Can you work these out from the drawing? Everything is in mm from the part's minimum corner. A direction names the side the tool comes from. Give positions to 0.01 mm unless a question says otherwise; leave off trailing zeros. Order: outer loops, then holes, each group sorted by start corner. A loop starts at its lowest first (then second) coordinate and runs counter-clockwise, first axis right, second up. Notation, with made-up numbers: (9.25, 25.25) - (22.25, 25.25) arc R21 ccw to (22.25, 32.25) - close; hole circle Ø6 at (21.5, 23). An arc over 180 degrees is marked (long way). Answer as a JSON object with one key per item and string values.
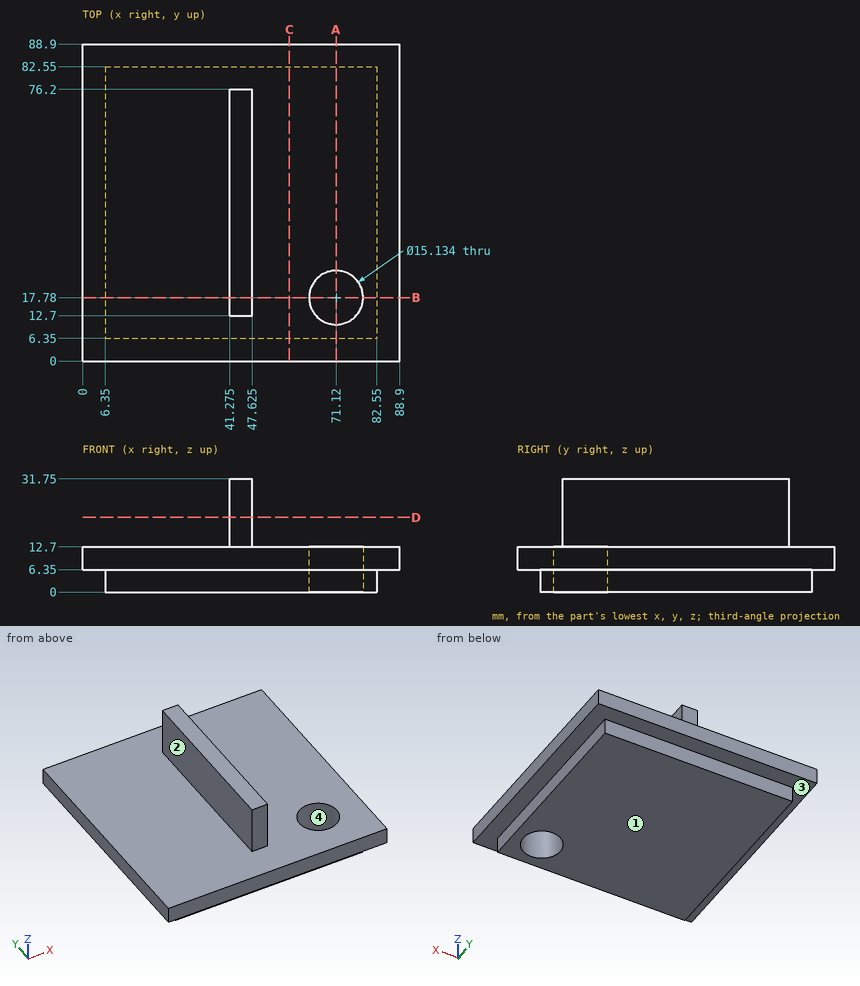
Q1. If we section it at B-B, the plane y = 17.78: Please give me the cut outline in (x, z) (3 decimals).
Recorded:
{"outline": "(0, 6.35) - (6.35, 6.35) - (6.35, 0) - (63.553, 0) - (63.553, 12.7) - (47.625, 12.7) - (47.625, 31.75) - (41.275, 31.75) - (41.275, 12.7) - (0, 12.7) - close; (78.687, 0) - (82.55, 0) - (82.55, 6.35) - (88.9, 6.35) - (88.9, 12.7) - (78.687, 12.7) - close"}
Q2. I'm going to push flat-ended pins straight in: pin 1 Ø1 at (y, z) = (14.5, 16.5) entering from -X (3 decimals); pin 2 Ø3 at (x, z) = (43, 17.5) entering from +Y; pin 3 Ø17.5 at (x, y) = (71.12, 17.78) entering from +Z. Where does each tip first touch, or does it pass through?
Recorded:
{"pin 1": "stops at x = 41.275", "pin 2": "stops at y = 76.2", "pin 3": "stops at z = 12.7"}
Q3. If we section it at A-A, the plane x = 71.12: Please give me the cut outline in (y, z), then the cut area to 3 significant figures.
Recorded:
{"outline": "(0, 6.35) - (6.35, 6.35) - (6.35, 0) - (10.21, 0) - (10.21, 12.7) - (0, 12.7) - close; (25.35, 0) - (82.55, 0) - (82.55, 6.35) - (88.9, 6.35) - (88.9, 12.7) - (25.35, 12.7) - close", "area": "856 mm^2"}
Q4. Which directions (+Z, -Z, +X, -X, +Y, -Y) give clear straight access to the entire face, cutting with the end or side of a thin tool? Please do the marked faces 1 and 2.
Recorded:
{"face 1": "-Z, +X, -X, +Y, -Y", "face 2": "+Z, -X, +Y, -Y"}
Q5. If we section it at D-D, the plane z = 21: Please give me the cut outline in (x, y) (3 decimals), then the cut area to 3 significant figures.
Recorded:
{"outline": "(41.275, 12.7) - (47.625, 12.7) - (47.625, 76.2) - (41.275, 76.2) - close", "area": "403 mm^2"}
Q6. If we section it at C-C, the plane x = 58: Please give me the cut outline in (y, z).
Recorded:
{"outline": "(0, 6.35) - (6.35, 6.35) - (6.35, 0) - (82.55, 0) - (82.55, 6.35) - (88.9, 6.35) - (88.9, 12.7) - (0, 12.7) - close"}
Q7. We'd pull the mould along Y, two halves only. Please class the marked faces 3 and 4: released by +Y, released by -Y, zero draft, split by the parting line, or undercut.
Recorded:
{"face 3": "zero draft", "face 4": "undercut"}
Q8. I need wall thicknesses on L1, parallel to Y at x = 71.12, z = 9.25; L2, parallel to Y at x = 71.12, z = 5.75; L3, parallel to Z at x = 54.5, y = 39. Which ranges of each line are inside material? Lowest first, please.
Recorded:
{"L1": "y = 0 to 10.21, 25.35 to 88.9", "L2": "y = 6.35 to 10.21, 25.35 to 82.55", "L3": "z = 0 to 12.7"}
